```python
from build123d import *

# Parameters (mm, degrees)
F1_DEPTH = 4
F2_R     = 89
F3_DEPTH = 2


with BuildPart() as f1:
    # F0 (on Top) → F1 (new body)
    with BuildSketch(Plane.XY):
        with BuildLine():
            Line((87.4, 0), (89.963485, -2.563485))
            ThreePointArc((89.963485, -2.563485), (2.563485, 89.963485), (-89.963485, 2.563485))
            Line((-89.963485, 2.563485), (-87.4, 0))
            ThreePointArc((-87.4, 0), (-64.224916, 59.278327), (-6.989929, 87.120037))
            ThreePointArc((-6.989929, 87.120037), (-4.715275, 86.334164), (-3.75, 84.129647))
            Line((-3.75, 84.129647), (-3.75, 79.15))
            ThreePointArc((-3.75, 79.15), (0, 75.4), (3.75, 79.15))
            Line((3.75, 79.15), (3.75, 84.129647))
            ThreePointArc((3.75, 84.129647), (4.715275, 86.334164), (6.989929, 87.120037))
            ThreePointArc((6.989929, 87.120037), (64.224916, 59.278327), (87.4, 0))
        make_face()
        with BuildLine():
            ThreePointArc((1.75, 79.15), (0, 77.4), (-1.75, 79.15))
            Line((-1.75, 79.15), (-1.75, 87.4))
            Line((-1.75, 87.4), (1.75, 87.4))
            Line((1.75, 87.4), (1.75, 79.15))
        make_face(mode=Mode.SUBTRACT)
    extrude(amount=F1_DEPTH)

    # F2 (on Top) → F3 (cut)
    with BuildSketch(Plane.XY):
        Circle(F2_R)
    extrude(amount=F3_DEPTH, mode=Mode.SUBTRACT)


solid = f1.part
```
Source: CAD feature listing. Evaluate the final solid. Frame: model axes, mm. A direction names the side the tool comes from. Give positions to 0.01 mm unless a question says otherwise; leave off trailing zeros. Loops run counter-clockwise (first coordinate to the right, second up) from the corner with the lowest first, then second, coordinate; pieces in that order, holes last. Notation, with made-up numbers: (86.25, -32.5) -> (133.25, -32.5) arc R21 cw to (133.25, -12.5) -> close; hole circle Ø5 at (5, 54.25). An arc over 180 degrees is marked (long way). Put each result on its own line as item: value. Start each with the question number.
1) Material intervals for probe 1 along X at (y, z) = (78.5, 3.3); probe 2 along X at (y, z) = (32.5, 2.3); probe 3 along X at (y, z) = (49.5, 2.1), sorted ascending.
2) Contact query for flat-ended pins moving along their axis: P1, Ø0.6, axis at x = 0.5, z = 2.5, coming from the -Y side; P2, Ø1, axis at y = 81.5, z = 3.5, coming from the -X side; P3, Ø0.6, axis at y = 82, z = 3, coming from the +X side; P4, Ø8, axis at x = -32.5, y = 76.5, coming from the -Z side. Output: stop coordinate, or through.
3) Cut plane D-D (y = 28). Return loops of the section in (x, z).
4) Cut plane A-A (x = 0). Return loops of the section in (y, z).
5) Reachability of faces 4 (the face through (-7, 88, 2)), 5 (the face through (-64.84, 58.605, 2.986)) from +Z, -Z, +X, -X, +Y, -Y: full face, straight path, thin tool, end or side. Return the list, or none.
6) Cut plane C-C (y = 48). Return loops of the section in (x, z), then the cut area to 3 significant figures.
7) Draft query along X for faces 1 (the face through (63.6, 59.95, 2.99)), 2 (the face through (0, 89, 4)), 3 (the face through (4.541, 89.885, 1.972)). Return one class per face: released by +X, released by -X, zero draft, split by the parting line, or undercut.
Results are:
1. probe 1: x = -44.02 to -38.43, -3.69 to -1.62, 1.62 to 3.69, 38.43 to 44.02
1. probe 2: x = -83.93 to -81.13, 81.13 to 83.93
1. probe 3: x = -75.16 to -72.03, 72.03 to 75.16
2. P1: stops at y = 75.41
2. P2: stops at x = -39.23
2. P3: stops at x = 37.75
2. P4: passes through
3. outline: (-85.53, 0) -> (-84.48, 0) -> (-84.48, 2) -> (-82.79, 2) -> (-82.79, 4) -> (-85.53, 4) -> close; (82.79, 2) -> (84.48, 2) -> (84.48, 0) -> (85.53, 0) -> (85.53, 4) -> (82.79, 4) -> close
4. outline: (75.4, 2) -> (77.4, 2) -> (77.4, 4) -> (75.4, 4) -> close; (87.4, 2) -> (89, 2) -> (89, 0) -> (90, 0) -> (90, 4) -> (87.4, 4) -> close
5. face 4: -Z, -Y
5. face 5: +Z, -Z, -Y
6. outline: (-76.13, 0) -> (-74.95, 0) -> (-74.95, 2) -> (-73.04, 2) -> (-73.04, 4) -> (-76.13, 4) -> close; (73.04, 2) -> (74.95, 2) -> (74.95, 0) -> (76.13, 0) -> (76.13, 4) -> (73.04, 4) -> close
6. area: 17.1 mm2
7. face 1: undercut
7. face 2: zero draft
7. face 3: split by the parting line
